Geometry: final body of the model. Coordinates: model frame, mm. Coordinates: 2 decimals unless noted, no trailing zeros. Write each loop counter-clockwise with the first axis right and the second up, starting at its lowest first coordinate (ties: lowest second). Pieces come first, ordered by that corner, then holes. Notation, with made-up numbers: (27, -1) - (48, -1) arc R26 ccw to (48, 23) - close; hole circle Ø10 at (68, 5). An arc over 180 degrees is marked (long way). Put each result on its own line as item: value.
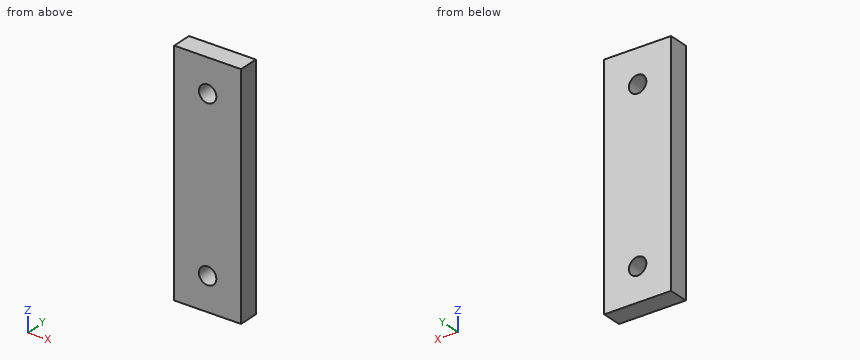
Autodesk Inventor part; units mm, degrees
ref_plane "YZ Plane" through (0, 0, 0) normal (1, 0, 0) x (0, 1, 0)
ref_plane "XZ Plane" through (0, 0, 0) normal (0, 1, 0) x (-1, 0, 0)
ref_plane "XY Plane" through (0, 0, 0) normal (0, 0, 1) x (1, 0, 0)
sketch "Sketch2" plane through (0, 0, 0) normal (0, 1, 0) x (-1, 0, 0)
  line L0 (0, 0) -> (-20, 0)
  line L1 (-20, 0) -> (-20, 70)
  line L2 (-20, 70) -> (0, 70)
  line L3 (0, 70) -> (0, 0)
  circle A0 centre (-10, 10) radius 2.6
  circle A1 centre (-10, 60) radius 2.6
  dimension "d76" = 20
  dimension "d78" = 10
  dimension "d79" = 50
  dimension "d80" = 10
  dimension "d81" = 5.2
  dimension "d82" = 10
extrude "Extrusion2" add sketch "Sketch2" along normal blind 6
properties part number "phone_holder_top_cap" material "Acrylic, Clear"
1. Section query D-D (z = 11.5). Return loops of the section in (x, y), then the cut area to 3 significant figures.
Answer below:
outline: (0, 0) - (7.88, 0) - (7.88, 6) - (0, 6) - close; (12.12, 0) - (20, 0) - (20, 6) - (12.12, 6) - close
area: 94.5 mm²
2. Section query B-B (z = 60). Return loops of the section in (x, y), then the cut area to 3 significant figures.
Answer below:
outline: (0, 0) - (7.4, 0) - (7.4, 6) - (0, 6) - close; (12.6, 0) - (20, 0) - (20, 6) - (12.6, 6) - close
area: 88.8 mm²
3. Section query C-C (y = 4). Return loops of the section in (x, z), then the cut area to 3 significant figures.
Answer below:
outline: (0, 0) - (20, 0) - (20, 70) - (0, 70) - close; hole circle Ø5.2 at (10, 10); hole circle Ø5.2 at (10, 60)
area: 1,360 mm²
4. Ray query, probe 1 along Z at (x, y) = (10, 1.8); probe 2 along X at (y, z) = (2.4, 59.5); probe 3 along X at (y, z) = (4.9, 61.5). Return the intervals inside material, ascending. Write a range as from..to.
Answer below:
probe 1: z = 0..7.4, 12.6..57.4, 62.6..70
probe 2: x = 0..7.45, 12.55..20
probe 3: x = 0..7.88, 12.12..20
5. Section query A-A (x = 10). Return loops of the section in (y, z), then the cut area to 3 significant figures.
Answer below:
outline: (0, 0) - (6, 0) - (6, 7.4) - (0, 7.4) - close; (0, 12.6) - (6, 12.6) - (6, 57.4) - (0, 57.4) - close; (0, 62.6) - (6, 62.6) - (6, 70) - (0, 70) - close
area: 358 mm²
